Autodesk Inventor part; units mm, degrees
ref_plane "YZ Plane" through (0, 0, 0) normal (1, 0, 0) x (0, 1, 0)
ref_plane "XZ Plane" through (0, 0, 0) normal (0, 1, 0) x (-1, 0, 0)
ref_plane "XY Plane" through (0, 0, 0) normal (0, 0, 1) x (1, 0, 0)
sketch "スケッチ1" plane through (0, 0, 0) normal (0, 0, 1) x (1, 0, 0)
  circle A0 centre (0, 0) radius 1.5
  dimension "d0" = 3
extrude "押し出し1" add sketch "スケッチ1" along normal blind 8
sketch "スケッチ2" plane through (0, 0, 8) normal (0, 0, 1) x (1, 0, 0)
  circle A0 centre (0, 0) radius 1.5
  circle A1 centre (0, 0) radius 3
  line L0 (0, 1.1547) -> (1, 0.5774)
  line L1 (1, 0.5774) -> (1, -0.5774)
  line L2 (1, -0.5774) -> (0, -1.1547)
  line L3 (0, -1.1547) -> (-1, -0.5774)
  line L4 (-1, -0.5774) -> (-1, 0.5774)
  line L5 (-1, 0.5774) -> (0, 1.1547)
  dimension "d3" = 6
  dimension "d6" = 2
extrude "押し出し2" add sketch "スケッチ2" against normal blind 1.7 contours A1
extrude "押し出し3" cut sketch "スケッチ2" against normal blind 1 contours L0 L1 L2 L3 L4 L5
chamfer "面取り1" distance 1.5 angle 45 1 edges at (-3, 0, 6.3)
properties part number "ねじ皿　m3-l8" material "鋼"
Build history of the part. All positions in model axes, mm. A direction names the side the tool comes from. Give positions to 0.01 mm unless a question says otherwise; leave off trailing zeros. Loops run counter-clockwise (first coordinate to the right, second up) from the corner with the lowest first, then second, coordinate; pieces in that order, holes last. Notation, with made-up numbers: (-10, 87.25) - (-6, 87.25) arc R8 ccw to (-6, 92.25) - close; hole circle Ø11 at (-9, 12). An arc over 180 degrees is marked (long way). Write item = value, one per line. Start each with the question number.
1) Pull direction X, two halves, no side cores. Call faces 3 (the flat face through (0.51, -0.86, 7.51)), 4 (the flat face through (0, 0, 0)), 5 (the cylindrical face through (-1.5, -0.07, 3.11)): +X half, -X half, draft (parallel to the pull), parting line (faces both ways), or undercut.
2) Tool access for faces 1 (the flat face through (0, 0, 7)), 2 (the flat face through (1.3, 0, 8)): list every direction of +Z, -Z, +X, -X, +Y, -Y with a clear straight run to the whole face (end or side of a thin tool).
3) Drop flat-ended pins along their axis: pin 1 Ø3 at (x, z) = (-1, 1) entering from -Y; pin 2 Ø3 at (y, z) = (1, 2.5) entering from -X; pin 3 Ø0.5 at (y, z) = (0, 7.5) entering from +X. Give the stop position or say it passes through.
4) Band-saw the part on B-B on z = 4. Give the cut face in (x, y).
5) Probe probe 1 along Y at (x, z) = (-0.05, 5.5); probe 2 along Z at (x, y) = (0, -0.2); probe 3 along Z at (x, y) = (2.2, -0.6). List the from-to ranges inside material, lowest first. Write a range as from..to.
Final values:
q1.face_3 = undercut
q1.face_4 = draft
q1.face_5 = parting line
q2.face_1 = +Z
q2.face_2 = +Z, +X, -X, +Y, -Y
q3.pin_1 = -1.5
q3.pin_2 = -1.5
q3.pin_3 = 2.95
q4.outline = circle Ø3 at (0, 0)
q5.probe_1 = -1.5..1.5
q5.probe_2 = 0..7
q5.probe_3 = 7.08..8
